The drawing under review shows one solid part. Ordinate dimensions are in mm from its lowest x, y, z. A direction names the side the tool comes from. Give positions to 0.01 mm unless a question says otherwise; leave off trailing zeros. Loops run counter-clockwise (first coordinate to the right, second up) from the corner with the lowest first, then second, coordinate; pieces in that order, holes last.
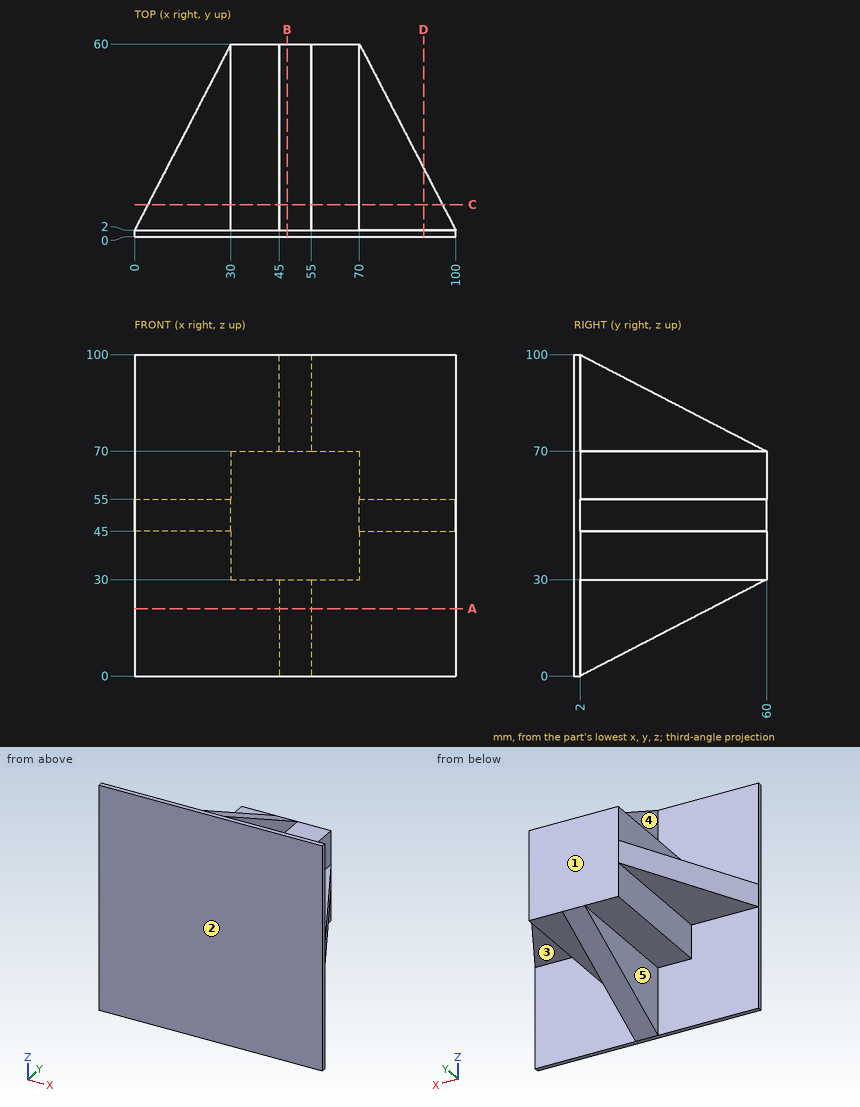
Item 1: Take a section at A-A on z = 21. Give the boundary of the cut face in (x, y).
Answer:
outline: (0, 0) - (100, 0) - (100, 2) - (55, 2) - (55, 42.6) - (45, 42.6) - (45, 2) - (0, 2) - close
Item 2: Take a section at D-D on x = 90. Give the boundary of the cut face in (y, z), and give its area (3 significant figures).
Answer:
outline: (0, 0) - (2, 0) - (2, 45) - (21.33, 45) - (21.33, 55) - (2, 55) - (2, 100) - (0, 100) - close
area: 393 mm2
Item 3: Tool access review of the marked faces 1, 2, 3, 4 and 5: name each direction out of +Z, -Z, +X, -X, +Y, -Y from which nothing blocks a thin tool from reaching the whole face with its end or side.
Answer:
face 1: +Z, -Z, +X, -X, +Y
face 2: +Z, -Z, +X, -X, -Y
face 3: -Z, +X, +Y
face 4: +Z, -X, +Y
face 5: -Z, -X, +Y
Item 4: Take a section at B-B on x = 47.5. Give the boundary of the cut face in (y, z), and give its area (3 significant figures).
Answer:
outline: (0, 0) - (2, 0) - (60, 30) - (60, 70) - (2, 100) - (0, 100) - close
area: 4,260 mm2
Item 5: For L1, parallel to X at y = 41.5, z = 58.5; L2, parallel to Y at x = 73, z = 63.5, list the stretches that pass through material, from the lowest coordinate up.
Answer:
L1: x = 30 to 70
L2: y = 0 to 2
Item 6: Clearance check with flat-ended pins moving along their axes: pin 1 Ø7.5 at (y, z) = (44.5, 60.5) entering from +X; pin 2 Ø9 at (x, y) = (11, 23.5) entering from +Z; pin 3 Ø16.5 at (y, z) = (41.5, 66) entering from -X; pin 4 Ø6 at (x, z) = (16, 51) entering from -Y. State where each tip first meets the part, or that it passes through.
Answer:
pin 1: stops at x = 70
pin 2: stops at z = 55
pin 3: stops at x = 30
pin 4: stops at y = 0
Item 7: Take a section at C-C on y = 10. Give the boundary of the cut face in (x, z).
Answer:
outline: (4.14, 45) - (30, 45) - (30, 30) - (45, 30) - (45, 4.14) - (55, 4.14) - (55, 30) - (70, 30) - (70, 45) - (95.86, 45) - (95.86, 55) - (70, 55) - (70, 70) - (55, 70) - (55, 95.86) - (45, 95.86) - (45, 70) - (30, 70) - (30, 55) - (4.14, 55) - close
